from build123d import *

# Parameters (mm, degrees)
SKETCH1_R           = 4.826
SKETCH1_R_2         = 3.3782
SKETCH1_R_3         = 2.5527
BOSS_EXTRUDE1_DEPTH = 4.7625


with BuildPart() as part:
    # Sketch1 → Boss-Extrude1 (new body)
    with BuildSketch(Plane(origin=(0, 4.7625, 0), x_dir=(1, 0, 0), z_dir=(0, 1, 0))):
        with BuildLine():
            Line((263.525, 25.4), (0, 25.4))
            ThreePointArc((0, 25.4), (-25.4, 0), (0, -25.4))
            Line((0, -25.4), (263.525, -25.4))
            ThreePointArc((263.525, -25.4), (288.925, 0), (263.525, 25.4))
        make_face()
        Circle(SKETCH1_R, mode=Mode.SUBTRACT)
        with Locations((263.525, 0)):
            Circle(SKETCH1_R, mode=Mode.SUBTRACT)
        with Locations((55.5625, -17.78)):
            Circle(SKETCH1_R_2, mode=Mode.SUBTRACT)
        with Locations((4.7625, -17.78)):
            Circle(SKETCH1_R_3, mode=Mode.SUBTRACT)
        with Locations((207.9625, 17.78)):
            Circle(SKETCH1_R_2, mode=Mode.SUBTRACT)
        with Locations((106.3625, -17.78)):
            Circle(SKETCH1_R_2, mode=Mode.SUBTRACT)
        with Locations((157.1625, -17.78)):
            Circle(SKETCH1_R_2, mode=Mode.SUBTRACT)
        with Locations((207.9625, -17.78)):
            Circle(SKETCH1_R_2, mode=Mode.SUBTRACT)
        with Locations((157.1625, 17.78)):
            Circle(SKETCH1_R_2, mode=Mode.SUBTRACT)
        with Locations((4.7625, 17.78)):
            Circle(SKETCH1_R_3, mode=Mode.SUBTRACT)
        with Locations((55.5625, 17.78)):
            Circle(SKETCH1_R_2, mode=Mode.SUBTRACT)
        with Locations((106.3625, 13.97)):
            Circle(SKETCH1_R, mode=Mode.SUBTRACT)
        with BuildLine():
            Line((166.6875, 11.43), (198.4375, 11.43))
            ThreePointArc((198.4375, 11.43), (200.68256403, 10.50006403), (201.6125, 8.255))
            Line((201.6125, 8.255), (201.6125, -8.255))
            ThreePointArc((201.6125, -8.255), (200.68256403, -10.50006403), (198.4375, -11.43))
            Line((198.4375, -11.43), (166.6875, -11.43))
            ThreePointArc((166.6875, -11.43), (164.44243597, -10.50006403), (163.5125, -8.255))
            Line((163.5125, -8.255), (163.5125, 8.255))
            ThreePointArc((163.5125, 8.255), (164.44243597, 10.50006403), (166.6875, 11.43))
        make_face(mode=Mode.SUBTRACT)
        with BuildLine():
            Line((122.526961018, 11.43), (147.6375, 11.43))
            ThreePointArc((147.6375, 11.43), (149.88256403, 10.50006403), (150.8125, 8.255))
            Line((150.8125, 8.255), (150.8125, -8.255))
            ThreePointArc((150.8125, -8.255), (149.88256403, -10.50006403), (147.6375, -11.43))
            Line((147.6375, -11.43), (115.8875, -11.43))
            ThreePointArc((115.8875, -11.43), (113.64243597, -10.50006403), (112.7125, -8.255))
            Line((112.7125, -8.255), (112.7125, -0.285714644))
            ThreePointArc((112.7125, -0.285714644), (113.087413196, 1.21099471), (114.123611111, 2.354232513))
            ThreePointArc((114.123611111, 2.354232513), (117.391826035, 5.39591887), (119.533542311, 9.313333333))
            ThreePointArc((119.533542311, 9.313333333), (120.693873913, 10.847376644), (122.526961018, 11.43))
        make_face(mode=Mode.SUBTRACT)
        with BuildLine():
            Line((72.306560788, 11.43), (90.198038982, 11.43))
            ThreePointArc((90.198038982, 11.43), (92.031126087, 10.847376644), (93.191457689, 9.313333333))
            ThreePointArc((93.191457689, 9.313333333), (95.333173965, 5.39591887), (98.601388889, 2.354232513))
            ThreePointArc((98.601388889, 2.354232513), (99.637586804, 1.21099471), (100.0125, -0.285714644))
            Line((100.0125, -0.285714644), (100.0125, -8.255))
            ThreePointArc((100.0125, -8.255), (99.08256403, -10.50006403), (96.8375, -11.43))
            Line((96.8375, -11.43), (72.306560788, -11.43))
            ThreePointArc((72.306560788, -11.43), (70.061496758, -10.50006403), (69.131560788, -8.255))
            Line((69.131560788, -8.255), (69.131560788, 8.255))
            ThreePointArc((69.131560788, 8.255), (70.061496758, 10.50006403), (72.306560788, 11.43))
        make_face(mode=Mode.SUBTRACT)
        with BuildLine():
            Line((20.635057548, 11.43), (46.0375, 11.43))
            ThreePointArc((46.0375, 11.43), (48.28256403, 10.50006403), (49.2125, 8.255))
            Line((49.2125, 8.255), (49.2125, -8.255))
            ThreePointArc((49.2125, -8.255), (48.28256403, -10.50006403), (46.0375, -11.43))
            Line((46.0375, -11.43), (20.635057548, -11.43))
            ThreePointArc((20.635057548, -11.43), (18.005907767, -10.034942816), (17.687192184, -7.075714286))
            ThreePointArc((17.687192184, -7.075714286), (19.05, 0), (17.687192184, 7.075714286))
            ThreePointArc((17.687192184, 7.075714286), (18.005907767, 10.034942816), (20.635057548, 11.43))
        make_face(mode=Mode.SUBTRACT)
        with BuildLine():
            Line((242.889942452, -11.43), (217.4875, -11.43))
            ThreePointArc((217.4875, -11.43), (215.24243597, -10.50006403), (214.3125, -8.255))
            Line((214.3125, -8.255), (214.3125, 8.255))
            ThreePointArc((214.3125, 8.255), (215.24243597, 10.50006403), (217.4875, 11.43))
            Line((217.4875, 11.43), (242.889942452, 11.43))
            ThreePointArc((242.889942452, 11.43), (245.519092233, 10.034942816), (245.837807816, 7.075714286))
            ThreePointArc((245.837807816, 7.075714286), (244.475, 0), (245.837807816, -7.075714286))
            ThreePointArc((245.837807816, -7.075714286), (245.519092233, -10.034942816), (242.889942452, -11.43))
        make_face(mode=Mode.SUBTRACT)
    extrude(amount=-BOSS_EXTRUDE1_DEPTH)


solid = part.part
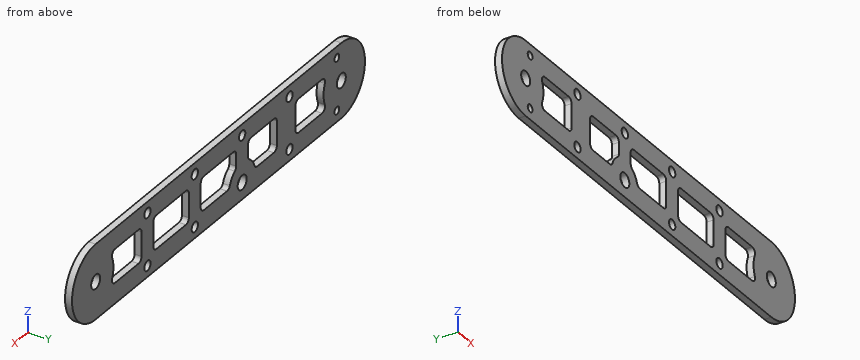
Can you work these out from the model? Positions are in its coordinate system, mm. Coordinates: 2 decimals unless noted, no trailing zeros. Loops run counter-clockwise (first coordinate to the right, second up) from the corner with the lowest first, then second, coordinate; pieces in that order, holes last. Notation, with made-up numbers: M -21,14.25 L 7,14.25 A16 cw 7,21.25 Z; hole C -24,53.25 d5. An arc over 180 degrees is marked long. Return JSON: item names as keys, results as strings. Group by question number.
Item 1: Imagine slicing it at C-C (y = 0.95). Give the number of separate pieces and of enclosed holes in the cut face, and give its area (3 significant figures).
Item 2: Imagine slicing it at B-B (z = 17.78). Please give me the cut outline in (x, y).
Item 3: If I drill on L1, parallel to X at y = 1.8, z = -5.5; L2, parallel to Z at x = 179, y = 1.2; L3, parallel to X at y = 1.2, z = 17.78, over which ranges is the centre line in solid material (lowest first)? Write a range as from..to.
Item 4: Imagine slicing it at A-A (x = 144). Please give me the cut outline in (y, z).
Item 5: I'm going to push flat-ended pins straight in: pin 1 Ø1.4 at (y, z) = (3, 0) entering from +X (3 decimals); pin 2 Ø1.4 at (y, z) = (1.5, 1) entering from -X; pin 3 Ø2 at (y, z) = (3.5, 12) entering from -X. Where does each tip first touch, or does it pass through?
Verdict:
{
 "1": {"separate pieces": "1", "enclosed holes": "17", "area": "11,200 mm^2"},
 "2": {"outline": "M -18.14,0 L 2.21,0 L 2.21,4.76 L -18.14,4.76 Z; M 7.32,0 L 52.18,0 L 52.18,4.76 L 7.32,4.76 Z; M 58.94,0 L 102.98,0 L 102.98,4.76 L 58.94,4.76 Z; M 109.74,0 L 153.78,0 L 153.78,4.76 L 109.74,4.76 Z; M 160.54,0 L 204.58,0 L 204.58,4.76 L 160.54,4.76 Z; M 211.34,0 L 281.66,0 L 281.66,4.76 L 211.34,4.76 Z"},
 "3": {"L1": "x = -24.8..18.24, 49.21..69.13, 95.25..117.47, 150.81..163.51, 201.61..214.31, 245.29..288.32", "L2": "z = -25.4..-11.43, 11.43..25.4", "L3": "x = -18.14..2.21, 7.32..52.18, 58.94..102.98, 109.74..153.78, 160.54..204.58, 211.34..281.66"},
 "4": {"outline": "M 0,-25.4 L 4.76,-25.4 L 4.76,-11.43 L 0,-11.43 Z; M 0,11.43 L 4.76,11.43 L 4.76,25.4 L 0,25.4 Z"},
 "5": {"pin 1": "stops at x = 288.925", "pin 2": "stops at x = -25.4", "pin 3": "stops at x = -22.89"}
}
